Work out the finished part from the listing and answer in its coordinate system (mm). Face numbers are marked on the shaded views. A direction names the side the tool comes from. Round coordinates to 2 decimals unless told otherwise and drop trailing zeros. Order: outer loops, then holes, each group sorted by start corner. A loop starts at its lowest first (then second) coordinate and runs counter-clockwise, first axis right, second up. Notation, with made-up numbers: M -12,36.25 L 17,36.25 A24 cw 17,58.25 Z; hole C -19.5,64.25 d3. An arc over 180 degrees is marked long. Return JSON: item names as keys, results as strings.
Autodesk Inventor part; units mm, degrees
ref_plane "YZ Plane" through (0, 0, 0) normal (1, 0, 0) x (0, 1, 0)
ref_plane "XZ Plane" through (0, 0, 0) normal (0, 1, 0) x (-1, 0, 0)
ref_plane "XY Plane" through (0, 0, 0) normal (0, 0, 1) x (1, 0, 0)
sketch "Sketch1" plane through (0, 0, 0) normal (0, 0, 1) x (1, 0, 0)
  line L0 (0, 110) -> (0, 0)
  line L1 (0, 0) -> (58, 0)
  line L2 (58, 0) -> (58, 8)
  line L3 (58, 8) -> (14, 110)
  line L4 (14, 110) -> (0, 110)
  dimension "d0" = 58
  dimension "d1" = 8
  dimension "d2" = 14
  dimension "d59" = 110
extrude "Extrusion1" add sketch "Sketch1" along normal blind 6.5
sketch "Sketch4" plane through (0, 0, 6.5) normal (0, 0, 1) x (1, 0, 0)
  line L0 (0, 110) -> (0, 0)
  line L1 (0, 0) -> (58, 0)
  line L2 (0, 64) -> (-11, 64)
  line L3 (-13, 66) -> (-13, 70)
  line L4 (-11, 72) -> (0, 72)
  line L5 (0, 72) -> (0, 64)
  line L6 (0, 87) -> (-11, 87)
  line L7 (-13, 89) -> (-13, 93)
  line L8 (-11, 95) -> (0, 95)
  line L9 (0, 95) -> (0, 87)
  line L10 (19, 0) -> (27, 0)
  line L11 (27, 0) -> (27, -4.5)
  line L12 (25, -6.5) -> (21, -6.5)
  line L13 (19, -4.5) -> (19, 0)
  line L14 (42, 0) -> (50, 0)
  line L15 (50, 0) -> (50, -4.5)
  line L16 (48, -6.5) -> (44, -6.5)
  line L17 (42, -4.5) -> (42, 0)
  arc A0 (-11, 95) -> (-13, 93) centre (-11, 93) ccw
  arc A1 (-13, 89) -> (-11, 87) centre (-11, 89) ccw
  arc A2 (-11, 72) -> (-13, 70) centre (-11, 70) ccw
  arc A3 (-13, 66) -> (-11, 64) centre (-11, 66) ccw
  arc A4 (19, -4.5) -> (21, -6.5) centre (21, -4.5) ccw
  arc A5 (25, -6.5) -> (27, -4.5) centre (25, -4.5) ccw
  arc A6 (42, -4.5) -> (44, -6.5) centre (44, -4.5) ccw
  arc A7 (48, -6.5) -> (50, -4.5) centre (48, -4.5) ccw
  line L18 (14, 110) -> (0, 110)
  dimension "d30" = 2
  dimension "d31" = 8
  dimension "d32" = 8
  dimension "d33" = 8
  dimension "d34" = 8
  dimension "d35" = 13
  dimension "d36" = 6.5
  dimension "d37" = 15
  dimension "d38" = 15
  dimension "d39" = 19
  dimension "d60" = 15
extrude "Extrusion3" add sketch "Sketch4" against normal blind 6.5
sketch "Sketch5" plane through (0, 0, 6.5) normal (0, 0, 1) x (1, 0, 0)
  line L0 (0, 87) -> (0, 72)
  line L1 (0, 72) -> (-11, 72)
  line L2 (27, 0) -> (42, 0)
  line L3 (42, 0) -> (42, -4.5)
  line L4 (16.3, 81.75) -> (16.3, 77.25)
  line L5 (0, 77.25) -> (0, 81.75)
  line L6 (5, 84.25) -> (12.3, 84.25)
  line L7 (12.3, 74.75) -> (5, 74.75)
  line L8 (32.25, 16.3) -> (36.75, 16.3)
  line L9 (36.75, 0) -> (32.25, 0)
  line L10 (39.25, 12.3) -> (39.25, 5)
  line L11 (29.75, 5) -> (29.75, 12.3)
  line L12 (0, 81.75) -> (5, 81.75)
  line L13 (12.3, 81.75) -> (16.3, 81.75)
  line L14 (16.3, 77.25) -> (12.3, 77.25)
  line L15 (5, 77.25) -> (0, 77.25)
  line L16 (5, 74.75) -> (5, 77.25)
  line L17 (5, 81.75) -> (5, 84.25)
  line L18 (12.3, 84.25) -> (12.3, 81.75)
  line L19 (12.3, 77.25) -> (12.3, 74.75)
  line L20 (32.25, 0) -> (32.25, 5)
  line L21 (32.25, 12.3) -> (32.25, 16.3)
  line L22 (36.75, 16.3) -> (36.75, 12.3)
  line L23 (36.75, 5) -> (36.75, 0)
  line L24 (29.75, 12.3) -> (32.25, 12.3)
  line L25 (36.75, 12.3) -> (39.25, 12.3)
  line L26 (39.25, 5) -> (36.75, 5)
  line L27 (32.25, 5) -> (29.75, 5)
  point P0 (16.3, 79.5)
  point P1 (34.5, 16.3)
  dimension "d43" = 4.5
  dimension "d44" = 4.5
  dimension "d45" = 5
  dimension "d46" = 4
  dimension "d47" = 7.3
  dimension "d48" = 4
  dimension "d49" = 5
  dimension "d50" = 7.3
  dimension "d51" = 2.5
  dimension "d52" = 2.5
  dimension "d53" = 2.5
  dimension "d54" = 2.5
  dimension "d55" = 7.5
  dimension "d56" = 7.5
extrude "Extrusion4" cut sketch "Sketch5" against normal through all
properties part number "z_motor_brace"
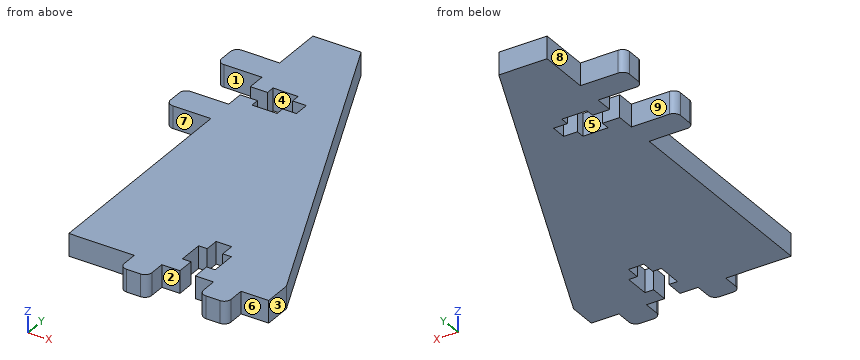
Item 1: The mould has two halves that part along Y. Classify the marked faces 1, 2, 3 and 4: pulls with the +Y half, pulls with the -Y half, needs draft (parallel to the pull), parting line crosses it, or undercut.
Output:
{"face 1": "undercut", "face 2": "pulls with the -Y half", "face 3": "needs draft", "face 4": "undercut"}
Item 2: Find section A-A (x = 7). Determine the outline of the cut face in (y, z).
Output:
{"outline": "M 0,0 L 74.75,0 L 74.75,6.5 L 0,6.5 Z; M 84.25,0 L 110,0 L 110,6.5 L 84.25,6.5 Z"}
Item 3: Each of these flat-tipped pins is pushed along its axis until it touches: pin 1 (2 mm diameter, centred on x = 38, z = 2.5, fed in from +Y); pin 2 (1.5 mm diameter, centred on x = 50, z = 2.5, fed in from +Y); pin 3 (3.5 mm diameter, centred on y = -2.5, z = 4, fed in from +X). Where does it stop, or does it pass through?
Output:
{"pin 1": "stops at y = 56.68", "pin 2": "stops at y = 28.28", "pin 3": "stops at x = 50"}
Item 4: Find section C-C (y = 26). Determine the outline of the cut face in (x, z), plus the area to 3 significant figures.
Output:
{"outline": "M 0,0 L 50.24,0 L 50.24,6.5 L 0,6.5 Z", "area": "327 mm^2"}
Item 5: Find section D-D (y = 90.5). Determine the outline of the cut face in (x, z).
Output:
{"outline": "M -13,0 L 22.41,0 L 22.41,6.5 L -13,6.5 Z"}
Item 6: Consider line 1 along Y through (x, z) = (9, 2); line 2 along Y through (x, z) = (-4.5, 4.5); line 3 along Y through (x, z) = (36, 5.25). Determine where each line is inside the solid, lowest interval first. Write a range as [from, to].
Output:
{"line 1": "y = [0, 74.75], [84.25, 110]", "line 2": "y = [64, 72], [87, 95]", "line 3": "y = [16.3, 59]"}
Item 7: Find section B-B (x = -2.5). Determine the outline of the cut face in (y, z), plus the area to 3 significant figures.
Output:
{"outline": "M 64,0 L 72,0 L 72,6.5 L 64,6.5 Z; M 87,0 L 95,0 L 95,6.5 L 87,6.5 Z", "area": "104 mm^2"}
Item 8: Which of the six approach directions +Z, -Z, +X, -X, +Y, -Y give full straight-line access (tool end or side, diameter ignored) to the marked faces 5, 6, 7, 8 and 9?
Output:
{"face 5": "+Z, -Z", "face 6": "+Z, -Z, +X, -Y", "face 7": "+Z, -Z, -X, -Y", "face 8": "+Z, -Z, -X, +Y", "face 9": "+Z, -Z, -X"}
